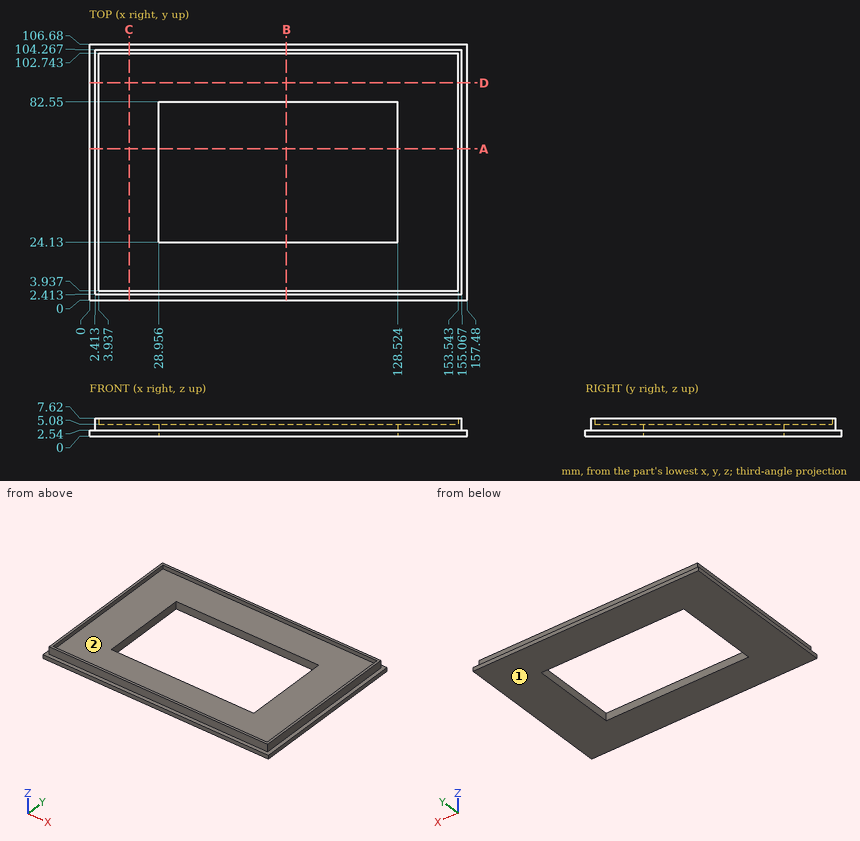
Answer from the drawing. Dimensions are ordinates in mm from the lowest x, y and z of the part. Round coordinates to 2 decimals unless told otherwise and drop trailing zeros. Loops run counter-clockwise (first coordinate to the right, second up) from the corner with the lowest first, then second, coordinate; pieces in that order, holes last.
1) A cutting plane is placed at B-B on x = 82. Determine the outline of the cut face in (y, z).
Outcome:
outline: (0, 0) - (24.13, 0) - (24.13, 5.08) - (3.94, 5.08) - (3.94, 7.62) - (2.41, 7.62) - (2.41, 2.54) - (0, 2.54) - close; (82.55, 0) - (106.68, 0) - (106.68, 2.54) - (104.27, 2.54) - (104.27, 7.62) - (102.74, 7.62) - (102.74, 5.08) - (82.55, 5.08) - close
2) A cutting plane is placed at C-C on x = 16.5. Determine the outline of the cut face in (y, z), plus the area to 3 significant figures.
Outcome:
outline: (0, 0) - (106.68, 0) - (106.68, 2.54) - (104.27, 2.54) - (104.27, 7.62) - (102.74, 7.62) - (102.74, 5.08) - (3.94, 5.08) - (3.94, 7.62) - (2.41, 7.62) - (2.41, 2.54) - (0, 2.54) - close
area: 537 mm2
3) For a pull along Y with two mould halves and no side action, classify the marked faces 1 and 2 as released by +Y, released by -Y, zero draft, split by the parting line, or undercut.
Outcome:
face 1: zero draft
face 2: undercut
4) A cutting plane is placed at D-D on y = 90.5. Determine the outline of the cut face in (x, z), plus the area to 3 significant figures.
Outcome:
outline: (0, 0) - (157.48, 0) - (157.48, 2.54) - (155.07, 2.54) - (155.07, 7.62) - (153.54, 7.62) - (153.54, 5.08) - (3.94, 5.08) - (3.94, 7.62) - (2.41, 7.62) - (2.41, 2.54) - (0, 2.54) - close
area: 795 mm2
5) Consider line 1 (X direction, y = 26, z = 6); line 2 (Y direction, x = 71.5, z = 2); line 3 (X direction, y = 42.5, z = 5). Determine where each line is inside the solid, lowest interval first.
Outcome:
line 1: x = 2.41 to 3.94, 153.54 to 155.07
line 2: y = 0 to 24.13, 82.55 to 106.68
line 3: x = 2.41 to 28.96, 128.52 to 155.07
6) Given P1, Ø2, axis at x = 16, y = 58, coming from the +Z side; P2, Ø1.5, axis at x = 52.5, z = 6, coming from the -Y side; P3, Ø1.5, axis at y = 57.5, z = 4.5, coming from the -X side, each flat-ended and moving along its own axis, determine where each tip first touches the part or whether it passes through.
Outcome:
P1: stops at z = 5.08
P2: stops at y = 2.41
P3: stops at x = 2.41
7) A cutting plane is placed at A-A on y = 63. Determine the outline of the cut face in (x, z), plus the area to 3 significant figures.
Outcome:
outline: (0, 0) - (28.96, 0) - (28.96, 5.08) - (3.94, 5.08) - (3.94, 7.62) - (2.41, 7.62) - (2.41, 2.54) - (0, 2.54) - close; (128.52, 0) - (157.48, 0) - (157.48, 2.54) - (155.07, 2.54) - (155.07, 7.62) - (153.54, 7.62) - (153.54, 5.08) - (128.52, 5.08) - close
area: 290 mm2
